Read the model definition and answer for the solid it produces. Units are mm, in the model's axes. Face numbers are marked on the shaded views. Round coordinates to 2 decimals unless told otherwise and drop trailing zeros. Write each loop counter-clockwise with the first axis right and the second up, starting at its lowest first coordinate (ties: lowest second). Pieces come first, ordered by that corner, then holes. Notation, with made-up numbers: (89.25, 29.5) -> (120.25, 29.5) arc R21 ccw to (120.25, 49.5) -> close; hole circle Ø1 at (-35, -23). An arc over 180 degrees is marked (long way). Return JSON: item names as keys, results as strings. Group by question number.
(1) Given pin 1 (2 mm diameter, centred on x = -0.5, z = -14.5, fed in from +Y); pin 2 (2 mm diameter, centred on x = 29.5, y = 3, fed in from +Z); pin 3 (3 mm diameter, centred on x = -29.5, y = 6, fed in from +Z), each flat-ended and moving along its own axis, determine where each tip first touches the part or whether it passes through.
(2) A cutting plane is placed at D-D on x = 0. State how many separate pieces and enclosed holes the cut face has, then the cut area to 3 significant figures.
(3) A cutting plane is placed at B-B on x = -15. Give the vertices of the cut face in (y, z), then the cut area to 3 significant figures.
(4) A cutting plane is placed at C-C on z = -15. Give the vertices of the cut face in (x, y).
(5) A cutting plane is placed at A-A on z = -30. Give the vertices of the cut face in (x, y).
(6) Straight lines are drawn through the part: line 1 (X direction, y = 2.25, z = 15); line 2 (X direction, y = 6.15, z = 15); line 3 (Z direction, x = 33, y = 5.25). For each, find the intervals that lie inside material, in ascending order.
(7) The mould has two halves that part along Z. Classify the marked faces 1, 2, 3 and 4: released by +Z, released by -Z, zero draft, split by the parting line, or undercut.
```python
from build123d import *

# Parameters (mm, degrees)
SKETCH1_W           = 75
SKETCH1_H           = 75
SKETCH1_R           = 6
SKETCH1_R_2         = 1.5
SKETCH1_R_3         = 1
BOSS_EXTRUDE1_DEPTH = 7
SKETCH2_R           = 3.25
CUT_EXTRUDE1_DEPTH  = 1.2
CHAMFER1_SIZE       = 10


with BuildPart() as part:
    # Sketch1 → Boss-Extrude1 (new body)
    with BuildSketch(Plane(origin=(0, 0, 0), x_dir=(1, 0, 0), z_dir=(0, 1, 0))):
        Rectangle(SKETCH1_W, SKETCH1_H)
        with Locations(Location((0, 0, 0), (0, 0, 270))):
            Circle(SKETCH1_R, mode=Mode.SUBTRACT)
        with Locations(Location((0, 15, 0), (0, 0, 270))):
            Circle(SKETCH1_R_2, mode=Mode.SUBTRACT)
        with Locations(Location((15, 0, 0), (0, 0, 270))):
            Circle(SKETCH1_R_2, mode=Mode.SUBTRACT)
        with Locations(Location((0, -15, 0), (0, 0, 270))):
            Circle(SKETCH1_R_2, mode=Mode.SUBTRACT)
        with Locations(Location((-15, 0, 0), (0, 0, 270))):
            Circle(SKETCH1_R_2, mode=Mode.SUBTRACT)
        with Locations(Location((-33.737040436, -9.03981274, 0), (0, 0, 270))):
            Circle(SKETCH1_R_2, mode=Mode.SUBTRACT)
        with Locations(Location((-33.737040436, 9.03981274, 0), (0, 0, 270))):
            Circle(SKETCH1_R_2, mode=Mode.SUBTRACT)
        with Locations(Location((-24.697227696, 24.697227696, 0), (0, 0, 270))):
            Circle(SKETCH1_R_2, mode=Mode.SUBTRACT)
        with Locations(Location((-9.03981274, 33.737040436, 0), (0, 0, 270))):
            Circle(SKETCH1_R_2, mode=Mode.SUBTRACT)
        with Locations(Location((9.03981274, 33.737040436, 0), (0, 0, 270))):
            Circle(SKETCH1_R_2, mode=Mode.SUBTRACT)
        with Locations(Location((24.697227696, 24.697227696, 0), (0, 0, 270))):
            Circle(SKETCH1_R_2, mode=Mode.SUBTRACT)
        with Locations(Location((33.737040436, 9.03981274, 0), (0, 0, 270))):
            Circle(SKETCH1_R_2, mode=Mode.SUBTRACT)
        with Locations(Location((33.737040436, -9.03981274, 0), (0, 0, 270))):
            Circle(SKETCH1_R_2, mode=Mode.SUBTRACT)
        with Locations(Location((24.697227696, -24.697227696, 0), (0, 0, 270))):
            Circle(SKETCH1_R_2, mode=Mode.SUBTRACT)
        with Locations(Location((9.03981274, -33.737040436, 0), (0, 0, 270))):
            Circle(SKETCH1_R_2, mode=Mode.SUBTRACT)
        with Locations(Location((-9.03981274, -33.737040436, 0), (0, 0, 270))):
            Circle(SKETCH1_R_2, mode=Mode.SUBTRACT)
        with Locations(Location((-24.697227696, -24.697227696, 0), (0, 0, 270))):
            Circle(SKETCH1_R_2, mode=Mode.SUBTRACT)
        with Locations(Location((0, 30, 0), (0, 0, 270))):
            Circle(SKETCH1_R_3, mode=Mode.SUBTRACT)
        with Locations(Location((25.980762114, 15, 0), (0, 0, 270))):
            Circle(SKETCH1_R_3, mode=Mode.SUBTRACT)
        with Locations(Location((25.980762114, -15, 0), (0, 0, 270))):
            Circle(SKETCH1_R_3, mode=Mode.SUBTRACT)
        with Locations(Location((0, -30, 0), (0, 0, 270))):
            Circle(SKETCH1_R_3, mode=Mode.SUBTRACT)
        with Locations(Location((-25.980762114, -15, 0), (0, 0, 270))):
            Circle(SKETCH1_R_3, mode=Mode.SUBTRACT)
        with Locations(Location((-25.980762114, 15, 0), (0, 0, 270))):
            Circle(SKETCH1_R_3, mode=Mode.SUBTRACT)
    extrude(amount=BOSS_EXTRUDE1_DEPTH)

    # Sketch2 → Cut-Extrude1 (cut)
    with BuildSketch(Plane(origin=(0, 7, 0), x_dir=(1, 0, 0), z_dir=(0, 1, 0))):
        with Locations(Location((0, 15, 0), (0, 0, 270))):
            Circle(SKETCH2_R)
        with Locations(Location((15, 0, 0), (0, 0, 270))):
            Circle(SKETCH2_R)
        with Locations(Location((0, -15, 0), (0, 0, 270))):
            Circle(SKETCH2_R)
        with Locations(Location((-15, 0, 0), (0, 0, 270))):
            Circle(SKETCH2_R)
    extrude(amount=-CUT_EXTRUDE1_DEPTH, mode=Mode.SUBTRACT)

    # Chamfer1
    chamfer1_edges = [part.edges().sort_by_distance(p)[0] for p in [
        (-37.5, 3.5, -37.5),
        (37.5, 3.5, -37.5),
        (37.5, 3.5, 37.5),
        (-37.5, 3.5, 37.5),
    ]]
    chamfer(chamfer1_edges, length=CHAMFER1_SIZE)


solid = part.part
```
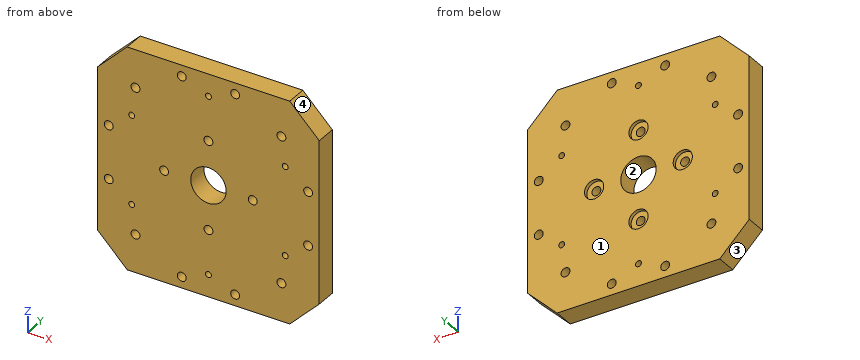
Checks:
{
 "1": {"pin 1": "stops at y = 5.8", "pin 2": "stops at z = 36.5", "pin 3": "stops at z = 37"},
 "2": {"separate pieces": "6", "enclosed holes": "0", "area": "363 mm^2"},
 "3": {"outline": "(0, -37.5) -> (7, -37.5) -> (7, -3.25) -> (5.8, -3.25) -> (5.8, -1.5) -> (0, -1.5) -> close; (0, 1.5) -> (5.8, 1.5) -> (5.8, 3.25) -> (7, 3.25) -> (7, 37.5) -> (0, 37.5) -> close", "area": "500 mm^2"},
 "4": {"outline": "(-37.5, 0) -> (-26.98, 0) -> (-26.98, 7) -> (-37.5, 7) -> close; (-24.98, 0) -> (-1.5, 0) -> (-1.5, 5.8) -> (-3.25, 5.8) -> (-3.25, 7) -> (-24.98, 7) -> close; (1.5, 0) -> (24.98, 0) -> (24.98, 7) -> (3.25, 7) -> (3.25, 5.8) -> (1.5, 5.8) -> close; (26.98, 0) -> (37.5, 0) -> (37.5, 7) -> (26.98, 7) -> close"},
 "5": {"outline": "(-35, 0) -> (-1, 0) -> (-1, 7) -> (-35, 7) -> close; (1, 0) -> (35, 0) -> (35, 7) -> (1, 7) -> close"},
 "6": {"line 1": "x = -37.5 to -26.98, -24.98 to -1.5, 1.5 to 24.98, 26.98 to 37.5", "line 2": "x = -37.5 to -26.98, -24.98 to -3.25, 3.25 to 24.98, 26.98 to 37.5", "line 3": "z = -32 to -10.35, -7.73 to 7.73, 10.35 to 32"},
 "7": {"face 1": "zero draft", "face 2": "undercut", "face 3": "released by -Z", "face 4": "released by +Z"}
}
